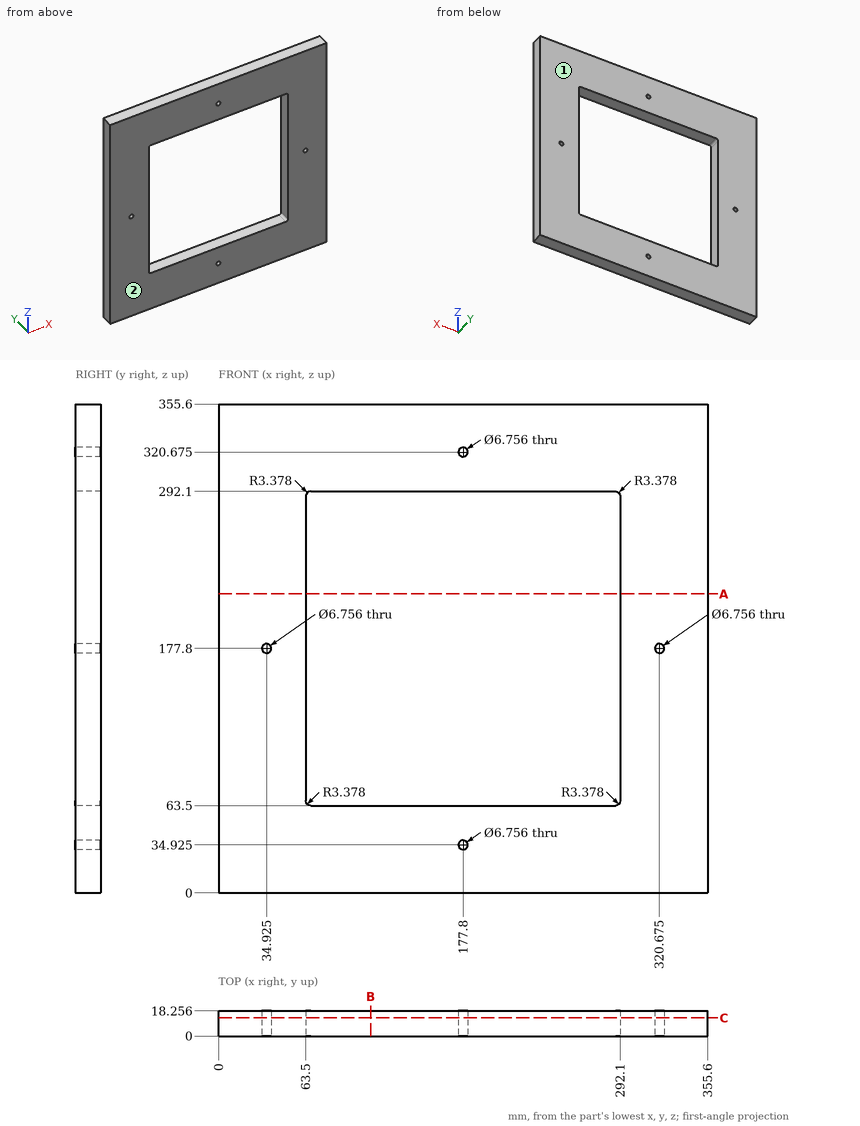
Part print with two shaded views. Sizes in mm from the minimum x, y, z corner. Round coordinates to 2 decimals unless told otherwise and drop trailing zeros. Order: outer loops, then holes, each group sorted by start corner. A loop starts at its lowest first (then second) coordinate and runs counter-clockwise, first axis right, second up. Notation, with made-up numbers: (-8.75, -31.75) -> (0.25, -31.75) arc R35 ccw to (0.25, 6.25) -> close; hole circle Ø10 at (-31, 9.5). An arc over 180 degrees is marked (long way). Use one line per item in the form item = value.
Item 1: Cut at C-C, the plane y = 13.25. Write the cut outline in (x, z) (1 decimal), and give its area (3 significant figures).
Returned:
outline = (0, 0) -> (355.6, 0) -> (355.6, 355.6) -> (0, 355.6) -> close; hole circle Ø6.8 at (34.9, 177.8); hole (63.5, 66.9) arc R3.4 ccw to (66.9, 63.5) -> (288.7, 63.5) arc R3.4 ccw to (292.1, 66.9) -> (292.1, 288.7) arc R3.4 ccw to (288.7, 292.1) -> (66.9, 292.1) arc R3.4 ccw to (63.5, 288.7) -> close; hole circle Ø6.8 at (177.8, 34.9); hole circle Ø6.8 at (177.8, 320.7); hole circle Ø6.8 at (320.7, 177.8)
area = 74,100 mm^2
Item 2: Drill centre line: line 1 (X direction, y = 4.25, z = 177.8). Where is it in solid material? Low to high.
Returned:
line_1 = 0 to 31.55, 38.3 to 63.5, 292.1 to 317.3, 324.05 to 355.6
Item 3: Cut at B-B, the plane x = 110.5. Write the cut outline in (y, z).
Returned:
outline = (0, 0) -> (18.26, 0) -> (18.26, 63.5) -> (0, 63.5) -> close; (0, 292.1) -> (18.26, 292.1) -> (18.26, 355.6) -> (0, 355.6) -> close
Item 4: Cut at A-A, the plane z = 217.5. Write the cut outline in (x, y), and give its area (3 significant figures).
Returned:
outline = (0, 0) -> (63.5, 0) -> (63.5, 18.26) -> (0, 18.26) -> close; (292.1, 0) -> (355.6, 0) -> (355.6, 18.26) -> (292.1, 18.26) -> close
area = 2,320 mm^2
Item 5: Pull direction Y, two halves, no side cores. Call the marked faces 1 and 2: released by +Y, released by -Y, zero draft, split by the parting line, or undercut.
Returned:
face_1 = released by +Y
face_2 = released by -Y
